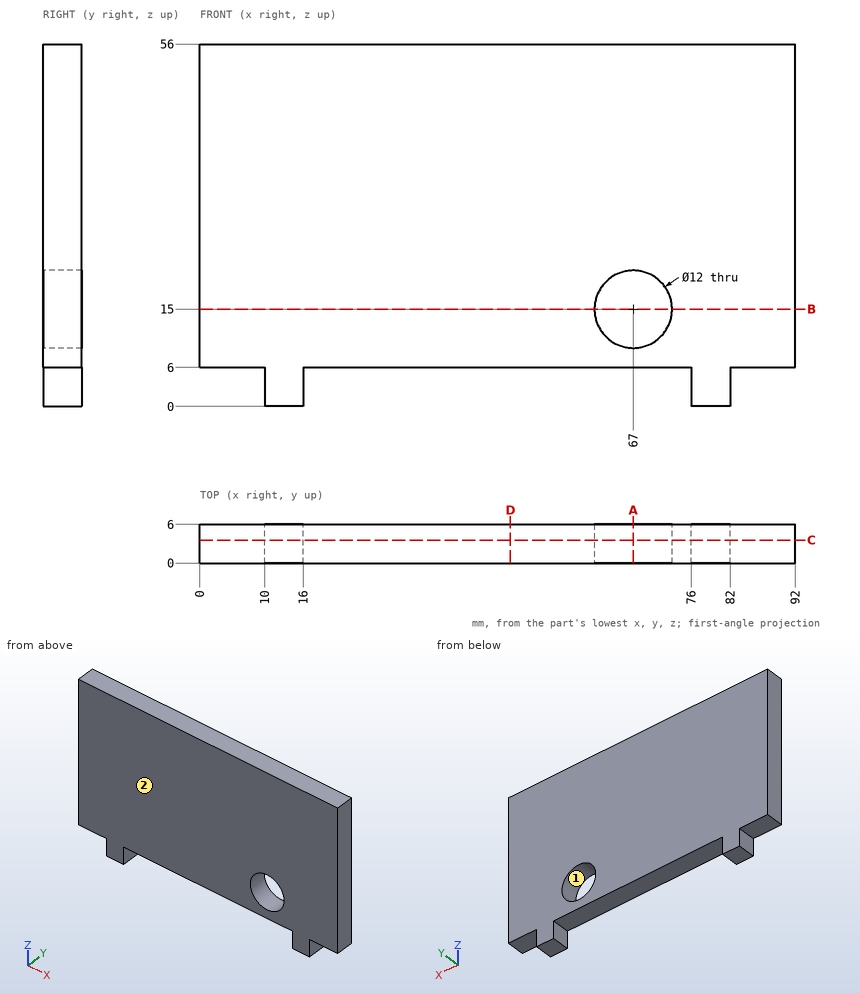
Answer from the drawing. Dimensions are ordinates in mm from the lowest x, y and z of the part. Round coordinates to 2 decimals unless told otherwise and drop trailing zeros. Write each loop counter-clockwise with the first axis right and the second up, starting at its lowest first coordinate (ties: lowest second). Pieces come first, ordered by that corner, then holes.
1. The part is cut by section D-D, the plane x = 48. Determine the outline of the cut face in (y, z), then the cut area to 3 significant figures.
2. The part is cut by section A-A, the plane x = 67. Determine the outline of the cut face in (y, z), then the cut area to 3 significant figures.
3. Determine the mould class of the marked faces 1 and 2 for opening direction X: pulls with the +X half, pulls with the -X half, needs draft (parallel to the pull), parting line crosses it, or undercut.
4. The part is cut by section C-C, the plane y = 3.55. Determine the outline of the cut face in (x, z).
5. The part is cut by section B-B, the plane z = 15. Determine the outline of the cut face in (x, y), then the cut area to 3 significant figures.
6. Given pin 1 Ø1 at (x, y) = (28.5, 1) entering from -Z; pin 2 Ø3 at (y, z) = (3.5, 2.5) entering from +X; pin 3 Ø1.8 at (y, z) = (2.5, 3.5) entering from -X; pin 4 Ø3 at (y, z) = (5, 46.5) entering from -X, each flat-ended and moving along its own axis, determine where each tip first touches the part or whether it passes through.
7. Straight lines are drawn through the part: L1, parallel to Z at x = 67, y = 3.5; L2, parallel to Z at x = 40.5, y = 3.7; L3, parallel to X at y = 3.55, z = 17.5. For each, find the intervals that lie inside material, in ascending order.
Values:
1. outline: (0, 6) - (6, 6) - (6, 56) - (0, 56) - close
1. area: 300 mm2
2. outline: (0, 6) - (6, 6) - (6, 9) - (0, 9) - close; (0, 21) - (6, 21) - (6, 56) - (0, 56) - close
2. area: 228 mm2
3. face 1: undercut
3. face 2: needs draft
4. outline: (0, 6) - (10, 6) - (10, 0) - (16, 0) - (16, 6) - (76, 6) - (76, 0) - (82, 0) - (82, 6) - (92, 6) - (92, 56) - (0, 56) - close; hole circle Ø12 at (67, 15)
5. outline: (0, 0) - (61, 0) - (61, 6) - (0, 6) - close; (73, 0) - (92, 0) - (92, 6) - (73, 6) - close
5. area: 480 mm2
6. pin 1: stops at z = 6
6. pin 2: stops at x = 82
6. pin 3: stops at x = 10
6. pin 4: stops at x = 0
7. L1: z = 6 to 9, 21 to 56
7. L2: z = 6 to 56
7. L3: x = 0 to 61.55, 72.45 to 92
